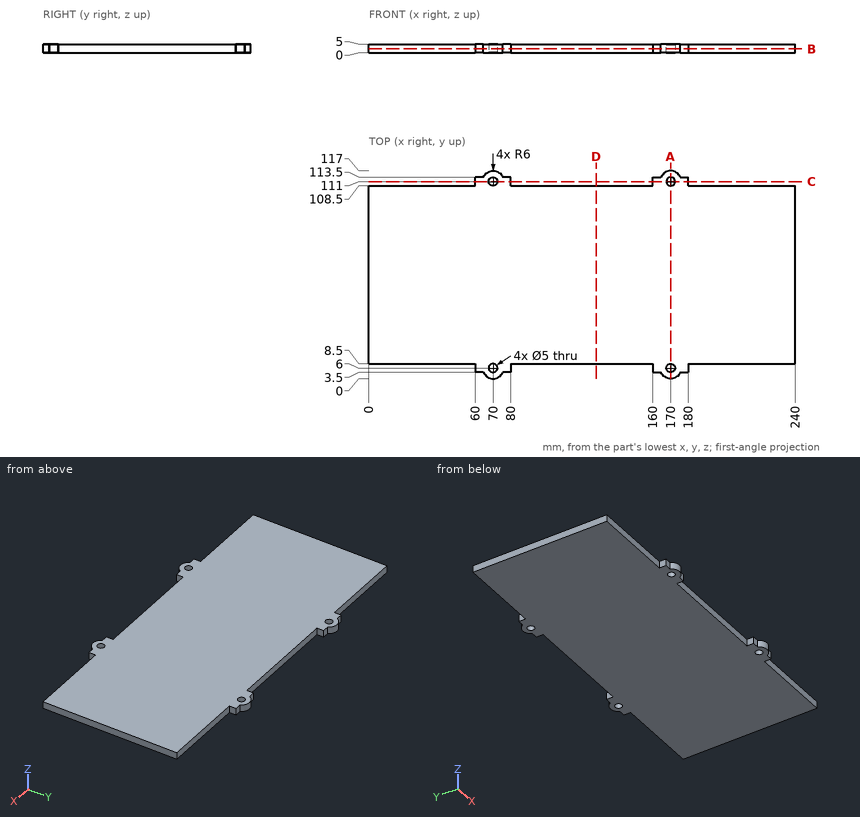
Here's the drawing with two shaded views (mm, measured from the low corner). I have some questions. Coordinates: 2 decimals unless noted, no trailing zeros. Loops run counter-clockwise (first coordinate to the right, second up) from the corner with the lowest first, then second, coordinate; pieces in that order, holes last. Notation, with made-up numbers: (-8, -8) - (27, -8) arc R13 ccw to (27, 8) - close; hole circle Ø7 at (10, 9.25). An arc over 180 degrees is marked (long way). Answer as CSV lines item,"result". Start each with the question number.
1) For pin 1 (4 mm diameter, centred on x = 170, y = 111, fed in from +Z); pin 2 (1.5 mm diameter, centred on y = 110.5, z = 1.5, fed in from -X); pin 3 (2.5 mm diameter, centred on x = 163, z = 1.5, fed in from +Y); pin 4 (1.5 mm diameter, centred on x = 214.5, z = 3.5, fed in from +Y), each with a flat end and sliding along its axis, tell me the tip position at first contact or that it passes through.
2) Suppose I cut it at C-C (y = 111). Please give me the cut outline in (x, z).
3) Suppose I cut it at A-A (x = 170). Please give me the cut outline in (y, z), plus the area to 3 significant figures.
4) Suppose I cut it at B-B (z = 2.25). Count the separate pieces of the cut face and the enclosed holes in it, plus the area to 3 significant figures.
5) I need wall thicknesses on line 1 (X direction, y = 6, z = 3.6); line 2 (Y direction, x = 170, z = 2.05); line 3 (X direction, y = 109.5, z = 0.7). Which ranges of each line are inside material? Lowest first, please. Write a range as from..to.
6) Suppose I cut it at D-D (x = 128). Please give me the cut outline in (y, z), plus the area to 3 significant figures.
Check result:
1,pin 1,"passes through"
1,pin 2,"stops at x = 60"
1,pin 3,"stops at y = 113.5"
1,pin 4,"stops at y = 108.5"
2,outline,"(60, 0) - (67.5, 0) - (67.5, 5) - (60, 5) - close; (72.5, 0) - (80, 0) - (80, 5) - (72.5, 5) - close; (160, 0) - (167.5, 0) - (167.5, 5) - (160, 5) - close; (172.5, 0) - (180, 0) - (180, 5) - (172.5, 5) - close"
3,outline,"(0, 0) - (3.5, 0) - (3.5, 5) - (0, 5) - close; (8.5, 0) - (108.5, 0) - (108.5, 5) - (8.5, 5) - close; (113.5, 0) - (117, 0) - (117, 5) - (113.5, 5) - close"
3,area,"535 mm²"
4,separate pieces,"1"
4,enclosed holes,"4"
4,area,"24,400 mm²"
5,line 1,"x = 60..67.5, 72.5..80, 160..167.5, 172.5..180"
5,line 2,"y = 0..3.5, 8.5..108.5, 113.5..117"
5,line 3,"x = 60..68, 72..80, 160..168, 172..180"
6,outline,"(8.5, 0) - (108.5, 0) - (108.5, 5) - (8.5, 5) - close"
6,area,"500 mm²"
